Autodesk Inventor part; units mm, degrees
ref_plane "YZ Plane" through (0, 0, 0) normal (1, 0, 0) x (0, 1, 0)
ref_plane "XZ Plane" through (0, 0, 0) normal (0, 1, 0) x (-1, 0, 0)
ref_plane "XY Plane" through (0, 0, 0) normal (0, 0, 1) x (1, 0, 0)
sketch "Boceto1" plane through (0, 0, 0) normal (0, 0, 1) x (1, 0, 0)
  line L0 (-32.5, -12.5) -> (32.5, -12.5)
  line L1 (32.5, -12.5) -> (32.5, 12.5)
  line L2 (32.5, 12.5) -> (-32.5, 12.5)
  line L3 (-32.5, 12.5) -> (-32.5, -12.5)
  line L4 (-32.5, -12.5) -> (32.5, 12.5) construction
  line L5 (32.5, -12.5) -> (-32.5, 12.5) construction
  circle A0 centre (-14.5, 0) radius 0.75
  circle A1 centre (5.5, 0) radius 0.75
  circle A2 centre (27.5, 0) radius 0.75
  circle A3 centre (20, 0) radius 2
  circle A4 centre (12.5, 0) radius 0.75
  circle A5 centre (20, 7.5) radius 0.75
  circle A6 centre (20, -7.5) radius 0.75
  point P0 (0, 0)
  dimension "d0" = 65
  dimension "d1" = 25
  dimension "d11" = 1.5
  dimension "d12" = 1.5
  dimension "d13" = 1.5
  dimension "d14" = 4
  dimension "d15" = 1.5
  dimension "d16" = 1.5
  dimension "d17" = 1.5
extrude "Extrusión1" add sketch "Boceto1" along normal blind 2
fillet "Empalme1" radius 12 1 edges at (32.5, 12.5, 1)
fillet "Empalme2" radius 12 1 edges at (32.5, -12.5, 1)
sketch "Boceto2" plane through (0, 0, 2) normal (0, 0, 1) x (1, 0, 0)
  point P0 (0, 0)
properties part number "laterales" material "Acero, galvanizado"
Verification items for the finished model (mm, model axes). Coordinates: 2 decimals unless noted, no trailing zeros. Write each loop counter-clockwise with the first axis right and the second up, starting at its lowest first coordinate (ties: lowest second). Pieces come first, ordered by that corner, then holes. Notation, with made-up numbers: (-24.75, -29.5) - (33.25, -29.5) arc R14 cw to (33.25, -3.5) - close; hole circle Ø9 at (85, -26). An arc over 180 degrees is marked (long way). One line per question, with ' | ' between items. Start each with the question number.
1. Section check B-B (z = 1.2). Enter the section's corners in (x, y), plus the area to 3 significant figures.
2. Section check A-A (x = -14.5). Enter the section's corners in (y, z).
3. Section check C-C (y = 7.5). Enter the section's corners in (x, z).
4. Draft check along X on faces 1 (the cylindrical face through (11.75, -0.03, 0.99)), 2 (the cylindrical face through (28.89, -9.08, 1.01)), 3 (the flat face through (-32.5, 0, 1)), 4 (the flat face through (0, 0, 0)). Enter one of: released by +X, released by -X, zero draft, split by the parting line, or undercut.
5. Gauge pin test, flat end, axial feed: P1, Ø1.7, axis at x = 20, y = 7.5, coming from the +Z side. Record the tip position at first contact, or that the pin passes through.
6. Material ranges on line 1 along Y through (x, z) = (5.5, 0.5); line 2 along Y through (x, z) = (20, 0.9); line 3 along X through (y, z) = (-7.75, 1.1), recorded low to high.
7. Section check D-D (y = -10). Enter the section's corners in (x, z).
Computed values:
1) outline: (-32.5, -12.5) - (20.5, -12.5) arc R12 ccw to (32.5, -0.5) - (32.5, 0.5) arc R12 ccw to (20.5, 12.5) - (-32.5, 12.5) - close; hole circle Ø1.5 at (-14.5, 0); hole circle Ø1.5 at (5.5, 0); hole circle Ø1.5 at (12.5, 0); hole circle Ø4 at (20, 0); hole circle Ø1.5 at (20, -7.5); hole circle Ø1.5 at (20, 7.5); hole circle Ø1.5 at (27.5, 0) | area: 1,540 mm²
2) outline: (-12.5, 0) - (-0.75, 0) - (-0.75, 2) - (-12.5, 2) - close; (0.75, 0) - (12.5, 0) - (12.5, 2) - (0.75, 2) - close
3) outline: (-32.5, 0) - (19.25, 0) - (19.25, 2) - (-32.5, 2) - close; (20.75, 0) - (30.25, 0) - (30.25, 2) - (20.75, 2) - close
4) face 1: undercut | face 2: released by +X | face 3: released by -X | face 4: zero draft
5) P1: z = 2
6) line 1: -12.5 to -0.75, 0.75 to 12.5 | line 2: -12.5 to -8.25, -6.75 to -2, 2 to 6.75, 8.25 to 12.5 | line 3: -32.5 to 19.29, 20.71 to 30.06
7) outline: (-32.5, 0) - (27.83, 0) - (27.83, 2) - (-32.5, 2) - close
